```python
from build123d import *

# Parameters (mm, degrees)
CROQUIS1_W              = 33.02
CROQUIS1_H              = 38.1
SALIENTE_EXTRUIR1_DEPTH = 1
CROQUIS2_R              = 0.635
CORTAR_EXTRUIR1_DEPTH   = 26.228606779


with BuildPart() as part:
    # Croquis1 → Saliente-Extruir1 (new body)
    with BuildSketch(Plane.XY):
        Rectangle(CROQUIS1_W, CROQUIS1_H)
    extrude(amount=SALIENTE_EXTRUIR1_DEPTH)

    # Croquis2 → Cortar-Extruir1 (cut, through all)
    with BuildSketch(Plane.XY.offset(1)):
        with Locations((-13.97, 15.24)):
            Circle(CROQUIS2_R)
        with Locations((-11.43, 15.24)):
            Circle(CROQUIS2_R)
        with Locations((-8.89, 15.24)):
            Circle(CROQUIS2_R)
        with Locations((-6.35, 15.24)):
            Circle(CROQUIS2_R)
        with Locations((-3.81, 15.24)):
            Circle(CROQUIS2_R)
        with Locations((-1.27, 15.24)):
            Circle(CROQUIS2_R)
        with Locations((1.27, 15.24)):
            Circle(CROQUIS2_R)
        with Locations((3.81, 15.24)):
            Circle(CROQUIS2_R)
        with Locations((6.35, 15.24)):
            Circle(CROQUIS2_R)
        with Locations((8.89, 15.24)):
            Circle(CROQUIS2_R)
        with Locations((11.43, 15.24)):
            Circle(CROQUIS2_R)
        with Locations((13.97, 15.24)):
            Circle(CROQUIS2_R)
        with Locations(Location((13.97, -15.24, 0), (0, 0, 180))):
            Circle(CROQUIS2_R)
        with Locations(Location((11.43, -15.24, 0), (0, 0, 180))):
            Circle(CROQUIS2_R)
        with Locations(Location((8.89, -15.24, 0), (0, 0, 180))):
            Circle(CROQUIS2_R)
        with Locations(Location((6.35, -15.24, 0), (0, 0, 180))):
            Circle(CROQUIS2_R)
        with Locations(Location((3.81, -15.24, 0), (0, 0, 180))):
            Circle(CROQUIS2_R)
        with Locations(Location((1.27, -15.24, 0), (0, 0, 180))):
            Circle(CROQUIS2_R)
        with Locations(Location((-1.27, -15.24, 0), (0, 0, 180))):
            Circle(CROQUIS2_R)
        with Locations(Location((-3.81, -15.24, 0), (0, 0, 180))):
            Circle(CROQUIS2_R)
        with Locations(Location((-6.35, -15.24, 0), (0, 0, 180))):
            Circle(CROQUIS2_R)
        with Locations(Location((-8.89, -15.24, 0), (0, 0, 180))):
            Circle(CROQUIS2_R)
        with Locations(Location((-11.43, -15.24, 0), (0, 0, 180))):
            Circle(CROQUIS2_R)
        with Locations(Location((-13.97, -15.24, 0), (0, 0, 180))):
            Circle(CROQUIS2_R)
    extrude(amount=-CORTAR_EXTRUIR1_DEPTH, mode=Mode.SUBTRACT)


solid = part.part
```
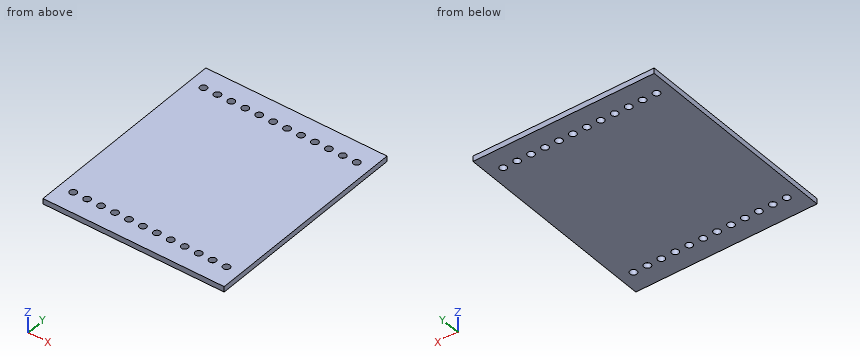
The listing builds one solid part. Answer for the finished solid, in the listing's coordinates (mm). Round coordinates to 2 decimals unless told otherwise and drop trailing zeros. Loops run counter-clockwise (first coordinate to the right, second up) from the corner with the lowest first, then second, coordinate; pieces in that order, holes last. Notation, with made-up numbers: (29.5, -1.75) -> (88.5, -1.75) arc R28 cw to (88.5, 21.25) -> close; hole circle Ø11 at (-26, 57). An arc over 180 degrees is marked (long way). Use one line per item in the form item = value.
1. Find the intervals of material crossed by probe 1 along Y at (x, z) = (-11.43, 0.5) (3 decimals); probe 2 along Y at (x, z) = (14.5, 0.95), in increasing order. Write a range as [from, to].
Answer key:
probe_1 = [-19.05, -15.875], [-14.605, 14.605], [15.875, 19.05]
probe_2 = [-19.05, -15.59], [-14.89, 14.89], [15.59, 19.05]
2. The part is cut by section B-B on z = 0.35. Give the number of separate pieces and of enclosed holes in the cut face, and give its area (3 significant figures).
Answer key:
separate_pieces = 1
enclosed_holes = 24
area = 1,230 mm²
3. The part is cut by section A-A on x = 1.27. Determine the outline of the cut face in (y, z) (3 decimals), and give its area (3 significant figures).
Answer key:
outline = (-19.05, 0) -> (-15.875, 0) -> (-15.875, 1) -> (-19.05, 1) -> close; (-14.605, 0) -> (14.605, 0) -> (14.605, 1) -> (-14.605, 1) -> close; (15.875, 0) -> (19.05, 0) -> (19.05, 1) -> (15.875, 1) -> close
area = 35.6 mm²
